```python
from build123d import *

# Parameters (mm, degrees)
SKETCH1_W                       = 80.1
SKETCH1_H                       = 20.27
SKETCH1_W_2                     = 12.4
SKETCH1_H_2                     = 6.4
BOSS_EXTRUDE1_DEPTH             = 1.75
SKETCH1_2_W                     = 12.4
SKETCH1_2_H                     = 6.4
BOSS_EXTRUDE2_DEPTH             = 14.7
BOSS_EXTRUDE3_REACH             = 85.961
SKETCH2_W                       = 7
SKETCH2_H                       = 4
BOSS_EXTRUDE3_DIRECTION_2_DEPTH = 13
SKETCH3_R                       = 2.4
BOSS_EXTRUDE4_DEPTH             = 18.55
SKETCH3_3_R                     = 2.4
BOSS_EXTRUDE5_DEPTH             = 17.2
FILLET1_R                       = 1.5


with BuildPart() as part:
    # Sketch1 → Boss-Extrude1 (new body)
    with BuildSketch(Plane(origin=(0, 0, 0), x_dir=(0, 0, -1), z_dir=(1, 0, 0))):
        with Locations((40.05, 10.135)):
            Rectangle(SKETCH1_W, SKETCH1_H)
        with Locations((40.05, 10.135)):
            Rectangle(SKETCH1_W_2, SKETCH1_H_2, mode=Mode.SUBTRACT)
    extrude(amount=BOSS_EXTRUDE1_DEPTH)

    # Sketch1<2> → Boss-Extrude2 (add)
    with BuildSketch(Plane(origin=(0, 0, 0), x_dir=(0, 0, -1), z_dir=(1, 0, 0))):
        with Locations((40.05, 10.135)):
            Rectangle(SKETCH1_2_W, SKETCH1_2_H)
    extrude(amount=BOSS_EXTRUDE2_DEPTH)

    # Boss-Extrude3: up to this plane
    boss_extrude3_end = Plane(origin=(1.75, 0, 0), z_dir=(1, 0, 0))
    # Sketch2 → Boss-Extrude3 (add, up to the surface)
    with BuildSketch(Plane(origin=(1.026942155, -0.861706784, 0), x_dir=(0, 0, -1), z_dir=(0.7660444431189771, -0.6427876096865406, 0)), mode=Mode.PRIVATE) as boss_extrude3_sk1:
        with Locations((15, 10.124878317)):
            Rectangle(SKETCH2_W, SKETCH2_H)
    boss_extrude3_tool1 = split(extrude(boss_extrude3_sk1.sketch, amount=-BOSS_EXTRUDE3_REACH, mode=Mode.PRIVATE), bisect_by=boss_extrude3_end, keep=Keep.BOTH, mode=Mode.PRIVATE)
    add(boss_extrude3_tool1.solids().sort_by_distance((7.535088, 6.8944, -15))[0])

    # Sketch2 → Boss-Extrude3 direction 2 (add)
    with BuildSketch(Plane(origin=(1.026942155, -0.861706784, 0), x_dir=(0, 0, -1), z_dir=(0.7660444431189771, -0.6427876096865406, 0))):
        with Locations((15, 10.124878317)):
            Rectangle(SKETCH2_W, SKETCH2_H)
    extrude(amount=BOSS_EXTRUDE3_DIRECTION_2_DEPTH)

    # Sketch3 → Boss-Extrude4 (add)
    with BuildSketch(Plane.ZY):
        with Locations(Location((-14.2, 12.55, 0), (0, 0, 180))):
            Circle(SKETCH3_R)
    extrude(amount=BOSS_EXTRUDE4_DEPTH)

    # Sketch3<3> → Boss-Extrude5 (add)
    with BuildSketch(Plane.ZY):
        with Locations(Location((-66.3, 12.55, 0), (0, 0, 180))):
            Circle(SKETCH3_3_R)
    extrude(amount=BOSS_EXTRUDE5_DEPTH)

    # Fillet1
    fillet1_edges = [part.edges().sort_by_distance(p)[0] for p in [
        (-18.55, 12.55, -11.8),
        (-17.2, 12.55, -63.9),
    ]]
    fillet(fillet1_edges, radius=FILLET1_R)


solid = part.part
```
Source: CAD feature listing. Evaluate the final solid. Frame: model axes, mm. A direction names the side the tool comes from. Give positions to 0.01 mm unless a question says otherwise; leave off trailing zeros. Loops run counter-clockwise (first coordinate to the right, second up) from the corner with the lowest first, then second, coordinate; pieces in that order, holes last. Notation, with made-up numbers: (-13, 65) -> (18, 65) arc R21 ccw to (18, 89) -> close; hole circle Ø1 at (15, -10). An arc over 180 degrees is marked (long way). Put each result on its own line as item: value. Start each with the question number.
1) Contact query for flat-ended pins moving along their axis: P1, Ø12, axis at x = 7.5, z = -25, coming from the -Y side; P2, Ø2, axis at y = 1, z = -39, coming from the -X side; P3, Ø0.5, axis at y = 12, z = -66.5, coming from the -X side. Output: stop coordinate, or through.
2) Material intervals for probe 1 along X at (y, z) = (1, -35); probe 2 along Z at (x, y) = (5.5, 7.5); probe 3 along Z at (x, y) = (10.5, 10.5), sorted ascending.
3) Reachability of faces 4 (the face through (8, 10, -46.25)), 5 (the face through (-17.2, 13, -66)), 6 (the face through (9, 6, -11.5)), 7 (the face through (-7.74, 13.469, -68.517)), 8 (the face through (8, 10, -33.85)) from +Z, -Z, +X, -X, +Y, -Y: full face, straight path, thin tool, end or side. Return the list, or none.
4) Draft query along X for faces 1 (the face through (17.51, -1.44, -14.95)), 2 (the face through (1, 10, -80.1)), 3 (the face through (8.878, 3.157, -14.951)). Return one class per face: released by +X, released by -X, zero draft, split by the parting line, or undercut.
5) Cut plane B-B (y = 4.25). Return loops of the section in (x, z).
6) Cut plane C-C (z = -20). Return loops of the section in (x, y).
Results are:
1. P1: stops at y = 0
1. P2: stops at x = 0
1. P3: stops at x = -17.2
2. probe 1: x = 0 to 1.75
2. probe 2: z = -46.25 to -33.85, -18.5 to -11.5
2. probe 3: z = -46.25 to -33.85
3. face 4: -Z, +X, +Y, -Y
3. face 5: -Z, -X, +Y, -Y
3. face 6: +Z, +X, +Y, -Y
3. face 7: -X
3. face 8: +X, +Y, -Y
4. face 1: released by +X
4. face 2: zero draft
4. face 3: undercut
5. outline: (0, -80.1) -> (1.75, -80.1) -> (1.75, 0) -> (0, 0) -> close; (7.58, -18.5) -> (13.8, -18.5) -> (13.8, -11.5) -> (7.58, -11.5) -> close
6. outline: (0, 0) -> (1.75, 0) -> (1.75, 20.27) -> (0, 20.27) -> close
